Can you work these out from the drawing? Everything is in mm from the part's minimum corner. A direction names the side the tool comes from. Coordinates: 2 decimals unless noted, no trailing zeros. Write each loop counter-clockwise with the first axis right and the second up, starting at its lowest first coordinate (ties: lowest second). Pieces come first, ordered by that corner, then holes. Notation, with made-up numbers: M 39,-32.75 L 76,-32.75 A5 cw 76,-27.75 Z; hole C -25,78 d1. An arc over 180 degrees is marked long. Write item = value, one per line.
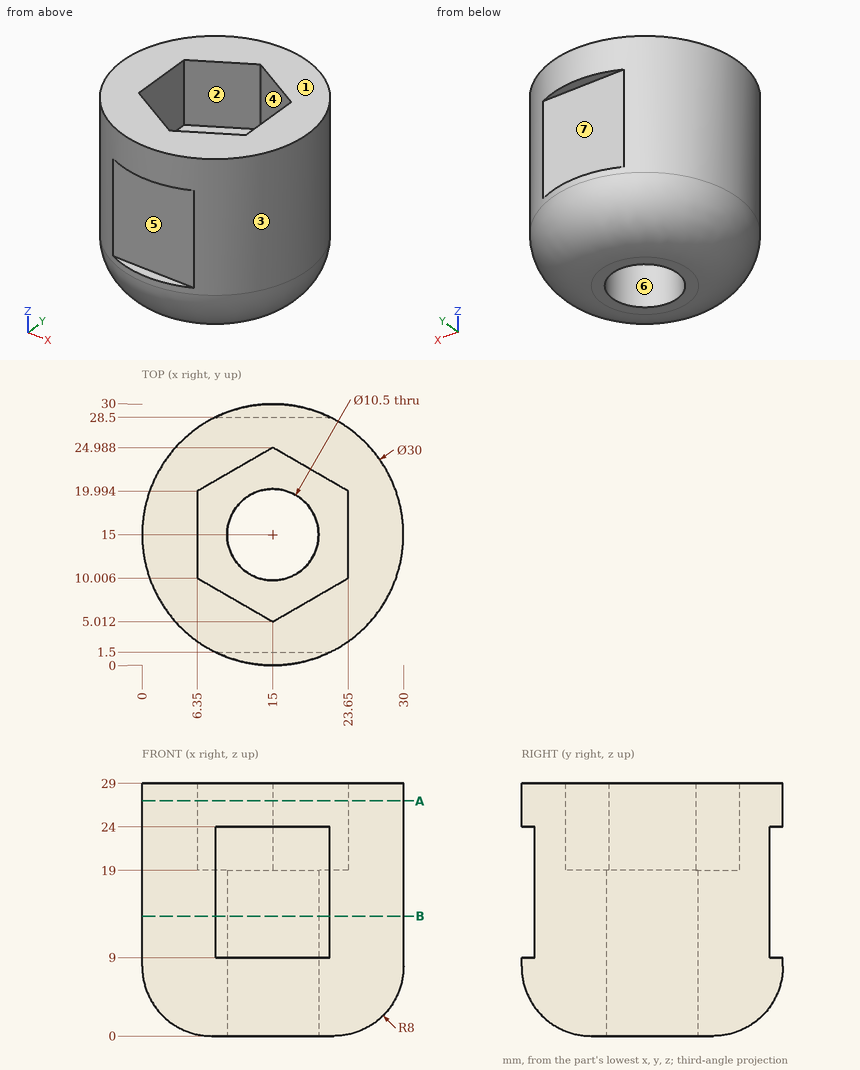
Item 1: For the marked faces 4, 5, 6 and 7, which set-ups out of +Z, -Z, +X, -X, +Y, -Y let a thin tool reach every point of the face, with its end or its side?
Numbers:
face_4 = +Z
face_5 = +X, -X, -Y
face_6 = +Z, -Z
face_7 = +X, -X, +Y
Item 2: I'm going to push flat-ended pins straight in: P1, Ø1.5, axis at y = 4.5, z = 24.5, coming from the +X side; P2, Ø8, axis at y = 17.5, z = 25, coming from the +X side; P3, Ø1, axis at x = 10.5, z = 15.5, coming from the +Y side; P4, Ø8.5, axis at x = 15, y = 15, coming from the +Z side. Where does each tip first touch, or does it pass through?
Numbers:
P1 = 26.4
P2 = 30
P3 = 28.5
P4 = through
Item 3: If I drill on line 1 along Y through (x, z) = (15, 12.5); line 2 along Y through (x, z) = (15, 8.5); line 3 along X through (y, z) = (14.75, 16), over which ranges is the centre line in solid material (lowest first)?
Numbers:
line_1 = 1.5 to 9.75, 20.25 to 28.5
line_2 = 0 to 9.75, 20.25 to 30
line_3 = 0 to 9.76, 20.24 to 30
Item 4: Imagine slicing it at B-B (z = 13.75). Write out the boundary of the cut face in (x, y).
Numbers:
outline = M 8.46,1.5 L 21.54,1.5 A15 ccw 21.54,28.5 L 8.46,28.5 A15 ccw Z; hole C 15,15 d10.5
Item 5: If we mould it in two halves opening along X, with no side actions, what happens to the marked faces 1, 2 and 3? For each: pulls with the +X half, pulls with the -X half, needs draft (parallel to the pull), parting line crosses it, or undercut.
Numbers:
face_1 = needs draft
face_2 = undercut
face_3 = parting line crosses it
Item 6: Imagine slicing it at A-A (z = 27). Write out the boundary of the cut face in (x, y).
Numbers:
outline = C 15,15 d30; hole M 6.35,10.01 L 15,5.01 L 23.65,10.01 L 23.65,19.99 L 15,24.99 L 6.35,19.99 Z
